```python
from build123d import *

# Parameters (mm, degrees)
SKETCH_3_R           = 2.825
CUT_EXTRUDE_2_DEPTH  = 35
SKETCH_16_W          = 5.008881277
SKETCH_16_H          = 1
EXTRUDE_2_DEPTH      = 30
SKETCH_19_W          = 0.959066555
SKETCH_19_H          = 0.511502163
EXTRUDE_3_DEPTH      = 30
SKETCH_24_W          = 26.827602514
SKETCH_24_H          = 4
CUT_EXTRUDE_8_DEPTH  = 9
EXTRUDE_1_DEPTH      = 2
EXTRUDE_1_DEPTH_BACK = 2
SKETCH_26_R          = 1.8
SKETCH_26_R_2        = 1
SKETCH_27_R          = 1.43
CUT_EXTRUDE_9_DEPTH  = 7
SKETCH_28_W          = 26.67763166
SKETCH_28_H          = 0.640570548
EXTRUDE_4_DEPTH      = 9
FILLET_1_R           = 10


with BuildPart() as part:
    # 草圖1 → 旋轉1 (revolve)
    with BuildSketch(Plane.XY, mode=Mode.PRIVATE) as revolve_1_sk:
        Polygon((0, 0), (0, 24.5), (4.87, 24.5), (10.87, 15), (15.87, 15), (21.87, 24.581141553), (26.74, 24.581141553), (26.74, 15), (36.74, 15), (36.74, 0), align=None)
    revolve(revolve_1_sk.sketch.rotate(Axis((-743.15639781, 0, 0), (1, 0, 0)), 90), axis=Axis((-743.15639781, 0, 0), (1, 0, 0)))

    # 草圖3 → 除料-伸長2 (cut)
    with BuildSketch(Plane(origin=(36.74, 0, 0), x_dir=(0, 0, -1), z_dir=(1, 0, 0))):
        Circle(SKETCH_3_R)
    extrude(amount=-CUT_EXTRUDE_2_DEPTH, mode=Mode.SUBTRACT)

    # 草圖16 → 填料-伸長2 (add)
    with BuildSketch(Plane(origin=(36.74, 0, 0), x_dir=(0, 0, -1), z_dir=(1, 0, 0))):
        with Locations((-0.105543204, 2.350977924)):
            Rectangle(SKETCH_16_W, SKETCH_16_H)
    extrude(amount=-EXTRUDE_2_DEPTH)

    # 草圖19 → 填料-伸長3 (add)
    with BuildSketch(Plane(origin=(36.74, 0, 0), x_dir=(0, 0, -1), z_dir=(1, 0, 0))):
        with Locations((-0.084116996, 2.673942601)):
            Rectangle(SKETCH_19_W, SKETCH_19_H)
    extrude(amount=-EXTRUDE_3_DEPTH)

    # 草圖24 → 除料-伸長8 (cut)
    with BuildSketch(Plane(origin=(36.74, 0, 0), x_dir=(0, 0, -1), z_dir=(1, 0, 0))):
        with Locations((1.262741112, 5.098242099)):
            Rectangle(SKETCH_24_W, SKETCH_24_H)
    extrude(amount=-CUT_EXTRUDE_8_DEPTH, mode=Mode.SUBTRACT)

    # 草圖26 → 伸長-薄件1 (add, two sides: drawn at the far end of the back side and taken through both)
    with BuildSketch(Plane.XY.offset(2).offset(-EXTRUDE_1_DEPTH_BACK)):
        with Locations((13.37, 16.023837481)):
            Circle(SKETCH_26_R)
        with Locations((13.37, 16.023837481)):
            Circle(SKETCH_26_R_2, mode=Mode.SUBTRACT)
    extrude(amount=EXTRUDE_1_DEPTH + EXTRUDE_1_DEPTH_BACK)

    # 草圖27 → 除料-伸長9 (cut)
    with BuildSketch(Plane(origin=(0, 12, 0), x_dir=(1, 0, 0), z_dir=(0, 1, 0))):
        with Locations(Location((31.545667046, 0, 0), (0, 0, 270))):
            Circle(SKETCH_27_R)
    extrude(amount=-CUT_EXTRUDE_9_DEPTH, mode=Mode.SUBTRACT)

    # 草圖28 → 填料-伸長4 (add)
    with BuildSketch(Plane(origin=(27.74, 0, 0), x_dir=(0, 0, -1), z_dir=(1, 0, 0))):
        with Locations((1.187755685, 3.418527373)):
            Rectangle(SKETCH_28_W, SKETCH_28_H)
    extrude(amount=EXTRUDE_4_DEPTH)

    # 圓角1
    # the kernel refuses this fillet: 10 mm, written as the material it takes off along each edge
    with BuildSketch(Plane(origin=(27.74, 3.738812647, -14.526571515), x_dir=(0, -1, 0), z_dir=(1, 0, 0))) as fillet_1_piece_1:
        with BuildLine():
            CenterArc((10, -3.521516765), FILLET_1_R, 159.381022137, 20.618977863)
            Line((0, -3.521516765), (-0.2, -3.521516765))
            Line((-0.2, -3.521516765), (-0.2, 0))
            Line((-0.2, 0), (0, 0.2))
            ThreePointArc((0, 0.2), (0.320285274, 0.2), (0.453381959, 0.070430335))
            Line((0.453381959, 0.070430335), (0.640570548, 0))
        make_face()
    extrude(amount=17.803791913, mode=Mode.SUBTRACT)


solid = part.part
```
CAD build for the part. Positions are in the model's coordinates, mm. A direction names the side the tool comes from. Coordinates: 2 decimals unless noted, no trailing zeros. Order: outer loops, then holes, each group sorted by start corner. A loop starts at its lowest first (then second) coordinate and runs counter-clockwise, first axis right, second up. Notation, with made-up numbers: M -37.5,52.25 L -11.5,52.25 A29 cw -11.5,72.25 Z; hole C 67,-39.5 d9. An arc over 180 degrees is marked long. Write each question's results on one line, items separated by ' | '. Start each with the question number.
Q1. Cut at A-A (x = 13.37). List the corners of the cut face in (y, z) (3 decimals).
Q2. Flat gauge pins, fed straight in: P1, Ø4.5, axis at x = 34, z = 4.5, coming from the +Y side; P2, Ø5, axis at x = 19.5, y = -14, coming from the +Z side; P3, Ø7, axis at x = 34.5, z = -6, coming from the -Y side. Where does each tip first touch, or does it go through?
Q3. Cut at C-C (x = 8). List the corners of the cut face in (y, z) (3 decimals), then the cut area to 3 significant figures.
Q4. Pull direction Z, two halves, no side cores. Call faces 6 (the flat face through (22, 1.851, 0)), 7 (the cylindrical face through (31.81, -12.65, 8.06)), 8 (the flat face through (27.74, 6, -1)), 9 (the flat face through (1.74, 0, 0)): +Z half, -Z half, draft (parallel to the pull), parting line (faces both ways), or undercut.
Q5. Cut at B-B (y = 0). List the corners of the cut face in (x, z) (3 decimals), then the cut area to 3 significant figures.
Q6. Drill centre lines: probe 1 along X at (y, z) = (10, 0); probe 2 along Y at (x, z) = (11, 0) (3 decimals); probe 3 along X at (y, z) = (6, 0). Where is each one in solid material? Low to high. Write a range as from..to.
Q7. Cut at D-D (x = 19). List the corners of the cut face in (y, z) (3 decimals), then the cut area to 3 significant figures.
Q8. Which spindle directions (+Z, -Z, +X, -X, +Y, -Y) get a long thin tool onto all of the face, cutting with end or side? Do faces 1 (the conical face through (10.58, 15.09, -3.35)), 2 (the flat face through (14, 17, 0)), 3 (the flat face through (14, 15, 4)), 4 (the cylindrical face through (2.47, -7.36, 23.37)), 5 (the cylindrical face through (32.177, 3.573, -12.819)). Say none if no direction does.
Found:
1) outline: M 14.457,4 A15 ccw long 15,0 L 15.024,0 L 15.024,4 Z; M 17.024,0 L 17.824,0 L 17.824,4 L 17.024,4 Z; hole M 1.851,-2.134 L 1.851,2.134 A2.825 ccw long Z
2) P1: y = 14.83 | P2: z = 20.73 | P3: y = -14.79
3) outline: C 0,0 d39.088; hole M 1.851,-2.134 L 1.851,2.134 A2.825 ccw long Z | area: 1,180 mm²
4) face 6: undercut | face 7: parting line | face 8: draft | face 9: undercut
5) outline: M 0,-24.5 L 4.87,-24.5 L 10.87,-15 L 15.87,-15 L 21.87,-24.581 L 26.74,-24.581 L 26.74,-15 L 36.74,-15 L 36.74,-2.825 L 1.74,-2.825 L 1.74,2.825 L 36.74,2.825 L 36.74,15 L 26.74,15 L 26.74,24.581 L 21.87,24.581 L 15.87,15 L 10.87,15 L 4.87,24.5 L 0,24.5 Z | area: 1,200 mm²
6) probe 1: 0..30.12, 32.98..36.74 | probe 2: -15..-2.825, 1.851..15 | probe 3: 0..27.74
7) outline: C 0,0 d39.996; hole M 1.851,-2.134 L 1.851,2.134 A2.825 ccw long Z | area: 1,230 mm²
8) face 1: none | face 2: -Z, +Y | face 3: +Z, +Y | face 4: -X | face 5: -Z, +X
